from build123d import *

# Parameters (mm, degrees)
F0_R      = 54
F0_R_2    = 28.575
F1_DEPTH  = 64
F2_R      = 11.1
F3_DEPTH  = 44
F6_DEPTH  = 22
F8_DEPTH  = 114.55193
F10_DEPTH = 10


with BuildPart() as f1:
    # F0 (on Front) → F1 (new body)
    with BuildSketch(Plane.XZ):
        Circle(F0_R)
        Circle(F0_R_2, mode=Mode.SUBTRACT)
    extrude(amount=F1_DEPTH)

    # F2 (on Front) → F3 (join)
    with BuildSketch(Plane.XZ):
        with BuildLine():
            ThreePointArc((33.941125, -42), (48.727922, -23.272078), (54, 0))
            ThreePointArc((54, 0), (48.727922, 23.272078), (33.941125, 42))
            ThreePointArc((33.941125, 42), (-54, 0), (33.941125, -42))
        make_face()
        with BuildLine():
            ThreePointArc((33.941125, 42), (48.727922, 23.272078), (54, 0))
            ThreePointArc((54, 0), (48.727922, -23.272078), (33.941125, -42))
            Line((33.941125, -42), (174, -42))
            Line((174, -42), (174, 42))
            Line((174, 42), (33.941125, 42))
        make_face()
        with Locations((89, 0)):
            Circle(F2_R, mode=Mode.SUBTRACT)
        with Locations((139, 0)):
            Circle(F2_R, mode=Mode.SUBTRACT)
    extrude(amount=F3_DEPTH)

    # F5 (on face) → F6 (cut)
    with BuildSketch(Plane.XZ.offset(44)):
        with BuildLine():
            Line((174, -26), (174, 26))
            Line((174, 26), (47.328638, 26))
            ThreePointArc((47.328638, 26), (54, 0), (47.328638, -26))
            Line((47.328638, -26), (174, -26))
        make_face()
    extrude(amount=-F6_DEPTH, mode=Mode.SUBTRACT)

    # F7 (on face) → F8 (cut)
    with BuildSketch(Plane.XY.offset(42)):
        Polygon((174, -32), (162, -44), (174, -44), align=None)
    extrude(amount=-F8_DEPTH, mode=Mode.SUBTRACT)

    # F9 (on face) → F10 (cut)
    with BuildSketch(Plane.XZ.offset(64)):
        with BuildLine():
            ThreePointArc((51.575188, 16), (0, 54), (-51.575188, 16))
            Line((-51.575188, 16), (-23.675528, 16))
            ThreePointArc((-23.675528, 16), (0, 28.575), (23.675528, 16))
            Line((23.675528, 16), (51.575188, 16))
        make_face()
        with BuildLine():
            Line((-23.675528, -16), (-51.575188, -16))
            ThreePointArc((-51.575188, -16), (0, -54), (51.575188, -16))
            Line((51.575188, -16), (23.675528, -16))
            ThreePointArc((23.675528, -16), (0, -28.575), (-23.675528, -16))
        make_face()
    extrude(amount=-F10_DEPTH, mode=Mode.SUBTRACT)


solid = f1.part
Could you check a few things on this model? Use its own coordinates, in mm. A direction names the side the tool comes from. Coordinates: 2 decimals unless noted, no trailing zeros. Loops run counter-clockwise (first coordinate to the right, second up) from the corner with the lowest first, then second, coordinate; pieces in that order, holes last.
1. Imagine slicing it at D-D (y = -27). Please give me the cut outline in (x, z).
2. For P1, Ø8, axis at x = 76, z = -33, coming from the -Y side; P2, Ø6, axis at y = -46, z = 32.5, coming from the +X side; P3, Ø3, axis at x = -41.5, y = -58, coming from the -Z side, each with a flat end and sliding along its axis, tell me the tip position at first contact or that it passes through.
3. We'd pull the mould along Z, two halves only. Please class faces 6 (the face through (27.255, -51.638, 8.583)), 7 (the face through (38, -59, -16)), 8 (the face through (105, -22, 42)), 9 (the face through (58, 0, 1)): released by +Z, released by -Z, zero draft, split by the parting line, or undercut.
4. I need wall thicknesses on L1, parallel to X at y = -11.75, z = 0; L2, parallel to Z at x = 69.5, y = -28.5; L3, parallel to Z at x = 89, y = -11. Which ranges of each line are inside material? Lowest first, please.
5. Imagine slicing it at A-A (y = -56.5). Please give me the cut outline in (x, z) (3 decimals).
6. Imagine slicing it at B-B (z = 0). Please give me the cut outline in (x, y) (3 decimals).
7. Imagine slicing it at C-C (x = 139). Please give me the cut outline in (y, z), and give its area (3 significant figures).
8. For faces 1 (the face through (-37, -59, -16)), 2 (the face through (110, -22, 0)), 3 (the face through (103, -22, -42)), 4 (the face through (-1, -54, 35)), 5 (the face through (127.91, -10.85, 0.49)), which set-ups out of +Z, -Z, +X, -X, +Y, -Y let a thin tool reach every point of the face, with its end or its side?
Computed values:
1. outline: (33.94, -42) - (174, -42) - (174, -26) - (47.33, -26) arc R54 ccw to (47.33, 26) - (174, 26) - (174, 42) - (33.94, 42) arc R54 ccw (long way) to start
2. P1: stops at y = -44
2. P2: stops at x = 163
2. P3: stops at z = -16
3. face 6: undercut
3. face 7: released by -Z
3. face 8: released by +Z
3. face 9: zero draft
4. L1: x = -54 to 77.9, 100.1 to 127.9, 150.1 to 174
4. L2: z = -42 to -26, 26 to 42
4. L3: z = -42 to -11.1, 11.1 to 42
5. outline: (-51.575, -16) - (-23.676, -16) arc R28.575 cw to (-23.676, 16) - (-51.575, 16) arc R54 ccw to start; (23.676, -16) - (51.575, -16) arc R54 ccw to (51.575, 16) - (23.676, 16) arc R28.575 cw to start
6. outline: (-54, -64) - (-28.575, -64) - (-28.575, -44) - (28.575, -44) - (28.575, -64) - (54, -64) - (54, -22) - (77.9, -22) - (77.9, 0) - (-54, 0) - close; (100.1, -22) - (127.9, -22) - (127.9, 0) - (100.1, 0) - close; (150.1, -22) - (174, -22) - (174, 0) - (150.1, 0) - close
7. outline: (-44, -42) - (0, -42) - (0, -11.1) - (-22, -11.1) - (-22, -26) - (-44, -26) - close; (-44, 26) - (-22, 26) - (-22, 11.1) - (0, 11.1) - (0, 42) - (-44, 42) - close
7. area: 2,060 mm2
8. face 1: -Z, +X, -X, -Y
8. face 2: +X, -Y
8. face 3: -Z, +X, +Y, -Y
8. face 4: +Z, +X, -X, -Y
8. face 5: +Y, -Y
